Could you check a few things on this model? Use its own coordinates, in mm. Give positions to 0.01 mm unless a question says otherwise; leave off trailing zeros. Order: outer loops, then holes, each group sorted by start corner. A loop starts at its lowest first (then second) coordinate and runs counter-clockwise, first axis right, second up. Notation, with made-up numbers: (18.25, -10.75) -> (66.25, -10.75) arc R14 ccw to (66.25, 15.25) -> close; hole circle Ø11 at (6, 32). An arc over 180 degrees is marked (long way). Write each question's results on one line, items separated by ' | '.
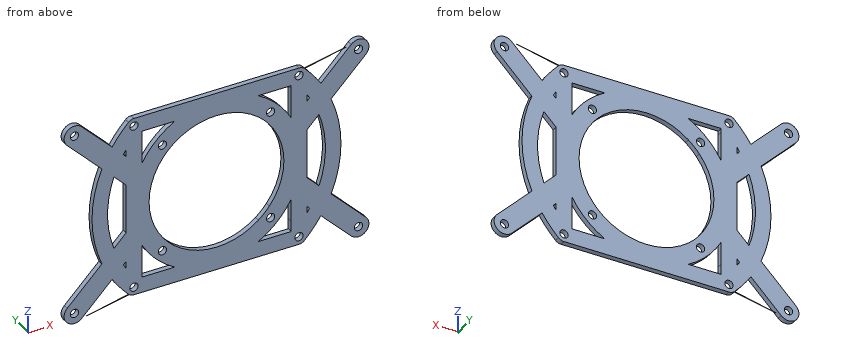
```python
from build123d import *

# Parameters (mm, degrees)
SKETCH1_R           = 1.6
BOSS_EXTRUDE1_DEPTH = 2
SKETCH2_R           = 48
SKETCH2_R_2         = 42
SKETCH2_R_3         = 1.6
BOSS_EXTRUDE2_DEPTH = 2
SKETCH3_R           = 1.6
BOSS_EXTRUDE3_DEPTH = 2
CUT_EXTRUDE1_DEPTH  = 10
FILLET1_R           = 3
BOSS_EXTRUDE4_DEPTH = 2
CUT_EXTRUDE2_START  = -10
SKETCH6_R           = 26
CUT_EXTRUDE2_DEPTH  = 10


with BuildPart() as part:
    # Sketch1 → Boss-Extrude1 (new body)
    with BuildSketch(Plane(origin=(0, 0, 0), x_dir=(1, 0, 0), z_dir=(0, 1, 0))):
        with BuildLine():
            Line((-51.943772875, 37.828427125), (-29.299283734, 15.183937983))
            ThreePointArc((-29.299283734, 15.183937983), (0, 33), (29.299283734, 15.183937983))
            Line((29.299283734, 15.183937983), (51.943772875, 37.828427125))
            ThreePointArc((51.943772875, 37.828427125), (57.600627125, 37.828427125), (57.600627125, 32.171572875))
            Line((57.600627125, 32.171572875), (32.280845123, 6.851790873))
            ThreePointArc((32.280845123, 6.851790873), (33, 0), (32.280845123, -6.851790873))
            Line((32.280845123, -6.851790873), (57.600627125, -32.171572875))
            ThreePointArc((57.600627125, -32.171572875), (57.600627125, -37.828427125), (51.943772875, -37.828427125))
            Line((51.943772875, -37.828427125), (29.299283734, -15.183937983))
            ThreePointArc((29.299283734, -15.183937983), (0, -33), (-29.299283734, -15.183937983))
            Line((-29.299283734, -15.183937983), (-51.943772875, -37.828427125))
            ThreePointArc((-51.943772875, -37.828427125), (-57.600627125, -37.828427125), (-57.600627125, -32.171572875))
            Line((-57.600627125, -32.171572875), (-32.280845123, -6.851790873))
            ThreePointArc((-32.280845123, -6.851790873), (-33, 0), (-32.280845123, 6.851790873))
            Line((-32.280845123, 6.851790873), (-57.600627125, 32.171572875))
            ThreePointArc((-57.600627125, 32.171572875), (-57.600627125, 37.828427125), (-51.943772875, 37.828427125))
        make_face()
        with Locations(Location((54.7722, 35, 0), (0, 0, 270))):
            Circle(SKETCH1_R, mode=Mode.SUBTRACT)
        with Locations(Location((-54.7722, 35, 0), (0, 0, 90))):
            Circle(SKETCH1_R, mode=Mode.SUBTRACT)
        with Locations(Location((54.7722, -35, 0), (0, 0, 90))):
            Circle(SKETCH1_R, mode=Mode.SUBTRACT)
        with Locations(Location((-54.7722, -35, 0), (0, 0, 270))):
            Circle(SKETCH1_R, mode=Mode.SUBTRACT)
        with Locations(Location((20.859650045, 20.859650045, 0), (0, 0, 270))):
            Circle(SKETCH1_R, mode=Mode.SUBTRACT)
        with Locations(Location((-20.859650045, 20.859650045, 0), (0, 0, 90))):
            Circle(SKETCH1_R, mode=Mode.SUBTRACT)
        with Locations(Location((20.859650045, -20.859650045, 0), (0, 0, 90))):
            Circle(SKETCH1_R, mode=Mode.SUBTRACT)
        with Locations(Location((-20.859650045, -20.859650045, 0), (0, 0, 270))):
            Circle(SKETCH1_R, mode=Mode.SUBTRACT)
        with BuildLine():
            Line((0, 4.242640687), (-16.140662024, 20.383302711))
            ThreePointArc((-16.140662024, 20.383302711), (0, 26), (16.140662024, 20.383302711))
            Line((16.140662024, 20.383302711), (0, 4.242640687))
        make_face(mode=Mode.SUBTRACT)
        with BuildLine():
            Line((0, -4.242640687), (-16.140662024, -20.383302711))
            ThreePointArc((-16.140662024, -20.383302711), (0, -26), (16.140662024, -20.383302711))
            Line((16.140662024, -20.383302711), (0, -4.242640687))
        make_face(mode=Mode.SUBTRACT)
        with BuildLine():
            Line((4.242640687, 0), (20.383302711, -16.140662024))
            ThreePointArc((20.383302711, -16.140662024), (26, 0), (20.383302711, 16.140662024))
            Line((20.383302711, 16.140662024), (4.242640687, 0))
        make_face(mode=Mode.SUBTRACT)
        with BuildLine():
            Line((-4.242640687, 0), (-20.383302711, -16.140662024))
            ThreePointArc((-20.383302711, -16.140662024), (-26, 0), (-20.383302711, 16.140662024))
            Line((-20.383302711, 16.140662024), (-4.242640687, 0))
        make_face(mode=Mode.SUBTRACT)
    extrude(amount=BOSS_EXTRUDE1_DEPTH)

    # Sketch2 → Boss-Extrude2 (add)
    with BuildSketch(Plane(origin=(0, 2, 0), x_dir=(1, 0, 0), z_dir=(0, 1, 0))):
        Circle(SKETCH2_R)
        Circle(SKETCH2_R_2, mode=Mode.SUBTRACT)
        with Locations(Location((31.819805153, 31.819805153, 0), (0, 0, 270))):
            Circle(SKETCH2_R_3, mode=Mode.SUBTRACT)
        with Locations(Location((-31.819805153, 31.819805153, 0), (0, 0, 270))):
            Circle(SKETCH2_R_3, mode=Mode.SUBTRACT)
        with Locations(Location((31.819805153, -31.819805153, 0), (0, 0, 270))):
            Circle(SKETCH2_R_3, mode=Mode.SUBTRACT)
        with Locations(Location((-31.819805153, -31.819805153, 0), (0, 0, 270))):
            Circle(SKETCH2_R_3, mode=Mode.SUBTRACT)
    extrude(amount=-BOSS_EXTRUDE2_DEPTH)

    # Sketch3 → Boss-Extrude3 (add)
    # profile 1 of 2: a face of its own
    with BuildSketch(Plane(origin=(0, 2, 0), x_dir=(1, 0, 0), z_dir=(0, 1, 0))):
        with BuildLine():
            Line((34.819811892, 31.819805153), (34.819811892, -31.819805153))
            ThreePointArc((34.819811892, -31.819805153), (31.819805153, -34.819811892), (28.819798415, -31.819805153))
            Line((28.819798415, -31.819805153), (28.819798415, 31.819805153))
            ThreePointArc((28.819798415, 31.819805153), (31.819805153, 34.819811892), (34.819811892, 31.819805153))
        make_face()
        with Locations(Location((31.819805153, -31.819805153, 0), (0, 0, 270))):
            Circle(SKETCH3_R, mode=Mode.SUBTRACT)
        with Locations(Location((31.819805153, 31.819805153, 0), (0, 0, 270))):
            Circle(SKETCH3_R, mode=Mode.SUBTRACT)
    # profile 2 of 2: a face of its own
    with BuildSketch(Plane(origin=(0, 2, 0), x_dir=(1, 0, 0), z_dir=(0, 1, 0))):
        with BuildLine():
            Line((-28.819798415, -31.819805153), (-28.819798415, 31.819805153))
            ThreePointArc((-28.819798415, 31.819805153), (-31.819805153, 34.819811892), (-34.819811892, 31.819805153))
            Line((-34.819811892, 31.819805153), (-34.819811892, -31.819805153))
            ThreePointArc((-34.819811892, -31.819805153), (-31.819805153, -34.819811892), (-28.819798415, -31.819805153))
        make_face()
        with Locations(Location((-31.819805153, 31.819805153, 0), (0, 0, 270))):
            Circle(SKETCH3_R, mode=Mode.SUBTRACT)
        with Locations(Location((-31.819805153, -31.819805153, 0), (0, 0, 270))):
            Circle(SKETCH3_R, mode=Mode.SUBTRACT)
    extrude(amount=-BOSS_EXTRUDE3_DEPTH)

    # Sketch4 → Cut-Extrude1 (cut)
    with BuildSketch(Plane(origin=(0, 2, 0), x_dir=(1, 0, 0), z_dir=(0, 1, 0))):
        Polygon((-28.819805153, 31.819805153), (-28.819805153, 24.740165209), (0, 38.846192425), (28.819805153, 24.740165209), (28.819805153, 31.819805153), (28.819805153, 53.488724091), (-28.819805153, 53.488724091), align=None)
        Polygon((28.819805153, -31.819805153), (28.819805153, -27.443703625), (0, -37.592318486), (-28.819805153, -27.443703625), (-28.819805153, -31.819805153), (-28.819805153, -57.678243433), (28.819805153, -57.678243433), align=None)
    extrude(amount=-CUT_EXTRUDE1_DEPTH, mode=Mode.SUBTRACT)

    # Fillet1
    # the kernel refuses this fillet: 3 mm, written as the material it takes off along each edge
    with BuildSketch(Plane(origin=(-28.819805153, -16.95161691, -38.385138152), x_dir=(0, 0, 1), z_dir=(0, 1, 0)), Plane(origin=(28.819805153, -16.95161691, 38.385138152), x_dir=(0, 0, -1), z_dir=(0, 1, 0))) as fillet1_piece_1:
        with BuildLine():
            CenterArc((6.565332998, -3), FILLET1_R, 90, 135)
            ThreePointArc((4.444012655, -5.121320344), (2.131461319, -2.639230371), (0, 0))
            Line((0, 0), (6.565332998, 0))
        make_face()
    extrude(amount=35.903233819, mode=Mode.SUBTRACT)
    with BuildSketch(Plane(origin=(-28.819805153, -16.95161691, 38.385138152), x_dir=(-0.755284934005079, 0, -0.6553965734308833), z_dir=(0, 1, 0)), Plane(origin=(28.819805153, -16.95161691, -38.385138152), x_dir=(0.7552849340050823, 0, 0.6553965734308795), z_dir=(0, 1, 0))) as fillet1_piece_2:
        with BuildLine():
            CenterArc((6.568751552, -2.99250738), FILLET1_R, 85.949727095, 135)
            Line((4.30289675, -4.9586971), (0, 0))
            ThreePointArc((0, 0), (3.390323382, 0.11988192), (6.780646764, 0))
        make_face()
    extrude(amount=35.903233819, mode=Mode.SUBTRACT)


with BuildPart() as boss_extrude4_tool:
    # Sketch5 → Boss-Extrude4 (new body)
    with BuildSketch(Plane(origin=(0, 2, 0), x_dir=(1, 0, 0), z_dir=(0, 1, 0))):
        Polygon((-31.819798415, 34.819811892), (31.819798415, 34.819811892), (29.753362448, 32.753375926), (28.819798415, 31.819811892), (28.819798415, 28.819811892), (0, 28.819811892), (-28.819798415, 28.819811892), (-28.819798415, 31.819811892), align=None)
        Polygon((-28.819798415, -31.819811892), (-31.819798415, -34.819811892), (31.819798415, -34.819811892), (29.753362448, -32.753375926), (28.819798415, -31.819811892), (28.819798415, -28.819811892), (0, -28.819811892), (-28.819798415, -28.819811892), align=None)
    extrude(amount=-BOSS_EXTRUDE4_DEPTH)


with BuildPart() as part_1:
    add(part.part)


with BuildPart() as part_2:
    # Boss-Extrude4: joined with boss_extrude4_tool
    add(part_1.part.fuse(boss_extrude4_tool.part, tol=0.00001))

    # Sketch6 → Cut-Extrude2 (cut)
    with BuildSketch(Plane(origin=(0, 2, 0), x_dir=(1, 0, 0), z_dir=(0, 1, 0)).offset(CUT_EXTRUDE2_START)):
        with Locations(Location((0, 0, 0), (0, 0, 270))):
            Circle(SKETCH6_R)
    extrude(amount=CUT_EXTRUDE2_DEPTH, mode=Mode.SUBTRACT)


solid = part_2.part
```
Q1. I'm going to push flat-ended pins straight in: pin 1 Ø1 at (x, y) = (-39.5, 1) entering from +Z; pin 2 Ø1 at (y, z) = (0.5, 22.5) entering from -X; pin 3 Ø1.1 at (y, z) = (1, 28) entering from -X. Where does each tip first touch, or does it pass through?
Here are the results:
pin 1: stops at z = 27.98 | pin 2: stops at x = -48.43 | pin 3: stops at x = -53.98
Q2. Suppose I cut it at D-D on z = 17.5. Please give me the cut outline in (x, y).
Here are the results:
outline: (-44.7, 0) -> (-28.82, 0) -> (-28.82, 2) -> (-44.7, 2) -> close; (-27.98, 0) -> (-19.23, 0) -> (-19.23, 2) -> (-27.98, 2) -> close; (19.23, 0) -> (27.98, 0) -> (27.98, 2) -> (19.23, 2) -> close; (28.82, 0) -> (44.7, 0) -> (44.7, 2) -> (28.82, 2) -> close
Q3. Suppose I cut it at C-C on x = -9. Please give me the cut outline in (y, z), and give its area (3 significant figures).
Here are the results:
outline: (0, -34.82) -> (2, -34.82) -> (2, -24.39) -> (0, -24.39) -> close; (0, 24.39) -> (2, 24.39) -> (2, 34.82) -> (0, 34.82) -> close | area: 41.7 mm²
Q4. I need wall thicknesses on line 1 along X through (y, z) = (1.8, -1); line 2 along X through (y, z) = (1.25, -12); line 3 along Z through (x, y) = (-20, 0.35). Which ranges of each line are inside material? Lowest first, please.
Here are the results:
line 1: x = -47.99 to -41.99, -34.82 to -25.98, 25.98 to 34.82, 41.99 to 47.99 | line 2: x = -46.48 to -40.25, -37.43 to -23.07, 23.07 to 37.43, 40.25 to 46.48 | line 3: z = -34.82 to -28.82, -26.25 to -22.21, -19.51 to -16.61, 16.61 to 19.51, 22.21 to 26.25, 28.82 to 34.82
Q5. Suppose I cut it at A-A on x = -24.5. Please give me the cut outline in (y, z).
Here are the results:
outline: (0, -34.82) -> (2, -34.82) -> (2, -28.82) -> (0, -28.82) -> close; (0, -22.11) -> (2, -22.11) -> (2, -8.7) -> (0, -8.7) -> close; (0, 8.7) -> (2, 8.7) -> (2, 22.11) -> (0, 22.11) -> close; (0, 28.82) -> (2, 28.82) -> (2, 34.82) -> (0, 34.82) -> close
